Drawing for the job (mm, zero at the part's lowest x, y, z). A direction names the side the tool comes from. Round coordinates to 2 decimals unless told otherwise and drop trailing zeros. Write each loop counter-clockwise with the first axis right and the second up, starting at its lowest first coordinate (ties: lowest second). Pieces come first, ordered by that corner, then holes. Notation, with made-up numbers: M 20,27 L 25,27 A15 ccw 25,38 Z; hole C 7.5,29.25 d5. An arc over 180 degrees is marked long. Use a Markdown table: item, result. Add a question column.
1) Which spindle directions (+Z, -Z, +X, -X, +Y, -Y) get a long thin tool onto all of the face, cutting with end or side? Do the marked faces 4 and 5. Say none if no direction does.
2) Wall check: probe 1 along Z at (x, y) = (2.9, 2.55); probe 2 along Z at (x, y) = (4.3, 3.45); probe 3 along X at (y, z) = (5, 0.5). Give the ranges that are in metal, low to high.
3) Slice it at D-D on x = 0.85. Write the cut outline in (y, z).
4) Two-plate mould, pull along X, no slides. Class the marked faces 1, 2 and 3: released by +X, released by -X, zero draft, split by the parting line, or undercut.
5) Drop flat-ended pins along their axis: P1, Ø0.6, axis at y = 3.5, z = 0, coming from the -X side; P2, Ø2, axis at y = 4, z = 4, coming from the -X side; P3, Ø2, axis at y = 3, z = 6, coming from the +X side. Give the stop position or say it passes through.
6) Slice it at A-A on x = 2.75. Write the cut outline in (y, z), plus the area to 3 significant figures.
7) Slice it at C-C on z = 7.5. Write the cut outline in (x, y), plus the area to 3 significant figures.
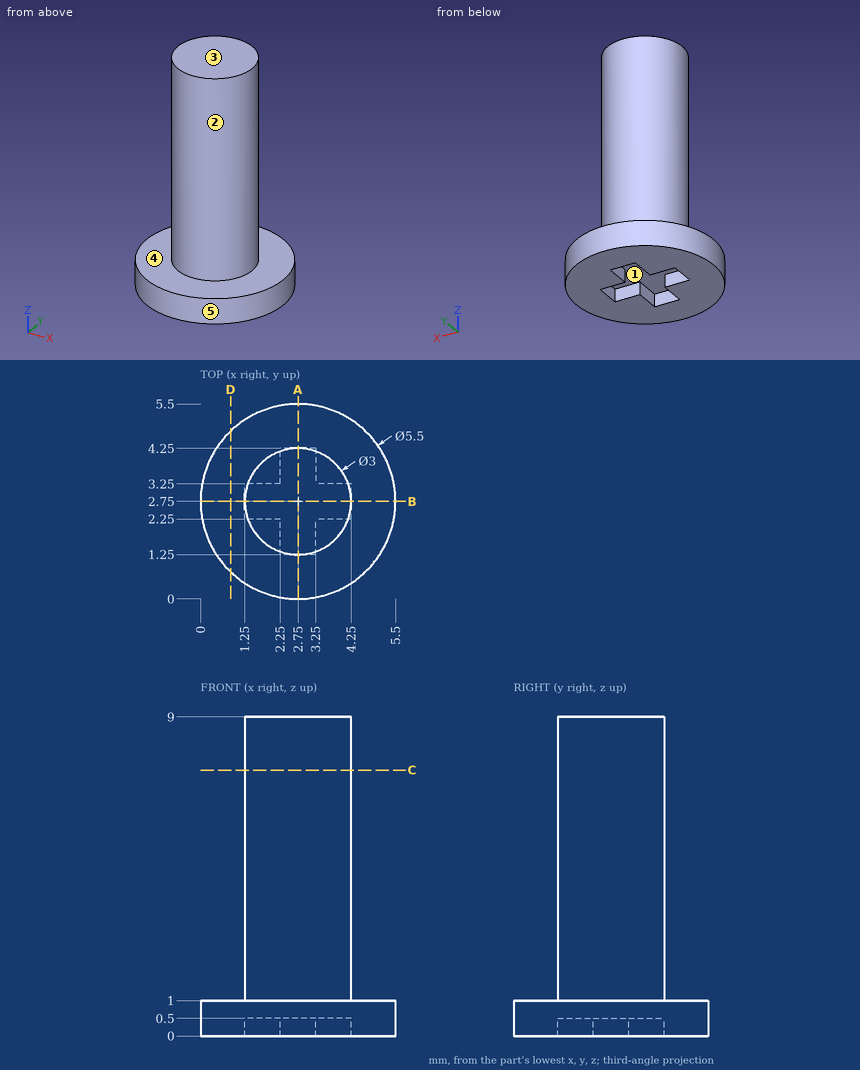
Entries:
| question | item | result |
|---|---|---|
| 1 | face 4 | +Z |
| 1 | face 5 | +Z, -Z |
| 2 | probe 1 | z = 0.5 to 9 |
| 2 | probe 2 | z = 0 to 1 |
| 2 | probe 3 | x = 1.17 to 4.33 |
| 3 | outline | M 0.76,0 L 4.74,0 L 4.74,1 L 0.76,1 Z |
| 4 | face 1 | undercut |
| 4 | face 2 | split by the parting line |
| 4 | face 3 | zero draft |
| 5 | P1 | stops at x = 0.04 |
| 5 | P2 | stops at x = 1.27 |
| 5 | P3 | stops at x = 4.25 |
| 6 | outline | M 0,0 L 1.25,0 L 1.25,0.5 L 4.25,0.5 L 4.25,0 L 5.5,0 L 5.5,1 L 4.25,1 L 4.25,9 L 1.25,9 L 1.25,1 L 0,1 Z |
| 6 | area | 28.0 mm^2 |
| 7 | outline | C 2.75,2.75 d3 |
| 7 | area | 7.07 mm^2 |
